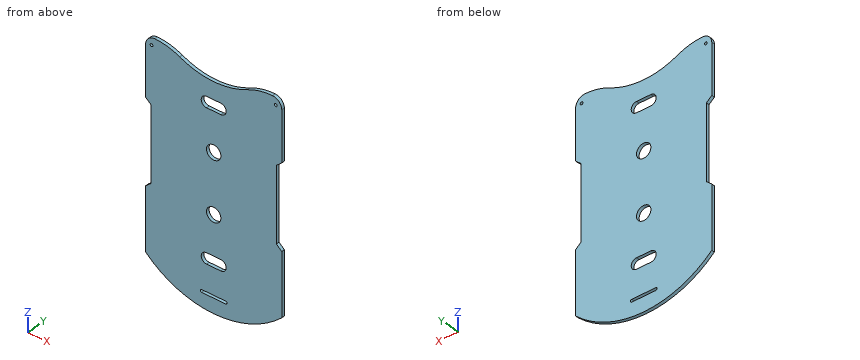
from build123d import *

# Parameters (mm, degrees)
CROQUIS1_R              = 8
CROQUIS1_R_2            = 1.55
SALIENTE_EXTRUIR1_DEPTH = 3.5


with BuildPart() as part:
    # Croquis1 → Saliente-Extruir1 (new body)
    with BuildSketch(Plane(origin=(0, 0, 0), x_dir=(1, 0, 0), z_dir=(0, 1, 0))):
        with BuildLine():
            Line((-75.83, 106.96), (-75.83, 36.96))
            Line((-75.83, 36.96), (-69.88, 31.76))
            Line((-69.88, 31.76), (-69.88, -51.39))
            Line((-69.88, -51.39), (-75.83, -56.59))
            Line((-75.83, -56.59), (-75.83, -112.67))
            ThreePointArc((-75.83, -112.67), (-72.813199846, -119.953199846), (-65.53, -122.97))
            ThreePointArc((-65.53, -122.97), (-51.316231926, -121.339014909), (-37.841336827, -116.530842982))
            ThreePointArc((-37.841336827, -116.530842982), (0, -107.730623626), (37.841336827, -116.530842982))
            ThreePointArc((37.841336827, -116.530842982), (51.316231926, -121.339014909), (65.53, -122.97))
            ThreePointArc((65.53, -122.97), (72.813199846, -119.953199846), (75.83, -112.67))
            Line((75.83, -112.67), (75.83, -56.59))
            Line((75.83, -56.59), (69.88, -51.39))
            Line((69.88, -51.39), (69.88, 31.76))
            Line((69.88, 31.76), (75.83, 36.96))
            Line((75.83, 36.96), (75.83, 106.96))
            ThreePointArc((75.83, 106.96), (0, 137.38), (-75.83, 106.96))
        make_face()
        with Locations(Location((0, 32.92, 0), (0, 0, 270))):
            Circle(CROQUIS1_R, mode=Mode.SUBTRACT)
        with Locations(Location((69.23, -114.59, 0), (0, 0, 270))):
            Circle(CROQUIS1_R_2, mode=Mode.SUBTRACT)
        with Locations(Location((0, -32.92, 0), (0, 0, 90))):
            Circle(CROQUIS1_R, mode=Mode.SUBTRACT)
        with Locations(Location((-69.23, -114.59, 0), (0, 0, 90))):
            Circle(CROQUIS1_R_2, mode=Mode.SUBTRACT)
        with BuildLine():
            Line((-7.895, -88.57), (7.895, -88.57))
            ThreePointArc((7.895, -88.57), (13.91, -82.555), (7.895, -76.54))
            Line((7.895, -76.54), (-7.895, -76.54))
            ThreePointArc((-7.895, -76.54), (-13.91, -82.555), (-7.895, -88.57))
        make_face(mode=Mode.SUBTRACT)
        with BuildLine():
            Line((-7.895, 88.57), (7.895, 88.57))
            ThreePointArc((7.895, 88.57), (13.91, 82.555), (7.895, 76.54))
            Line((7.895, 76.54), (-7.895, 76.54))
            ThreePointArc((-7.895, 76.54), (-13.91, 82.555), (-7.895, 88.57))
        make_face(mode=Mode.SUBTRACT)
        with BuildLine():
            Line((-13.415, 120.93), (13.415, 120.93))
            ThreePointArc((13.415, 120.93), (14.915, 119.43), (13.415, 117.93))
            Line((13.415, 117.93), (-13.415, 117.93))
            ThreePointArc((-13.415, 117.93), (-14.915, 119.43), (-13.415, 120.93))
        make_face(mode=Mode.SUBTRACT)
    extrude(amount=SALIENTE_EXTRUIR1_DEPTH)


solid = part.part
Source: CAD feature listing. Evaluate the final solid. Frame: model axes, mm. Give positions to 0.01 mm unless a question says otherwise; leave off trailing zeros. Write each loop counter-clockwise with the first axis right and the second up, starting at its lowest first coordinate (ties: lowest second). Pieces come first, ordered by that corner, then holes. Notation, with made-up numbers: M 7,21.5 L 25,21.5 A4 cw 25,26.5 Z; hole C 86,85 d6. An arc over 180 degrees is marked long. Answer as a JSON object with one key per item and string values.
Q1. Contact query for flat-ended pins moving along their axis: P1, Ø1.5, axis at x = 17, y = 3, coming from the -Z side; P2, Ø2, axis at x = 6.5, y = 2.5, coming from the +Z side; P3, Ø1.8, axis at y = 1, z = -4.5, coming from the -X side. Output: stop coordinate, or through.
Geometry check:
{"P1": "stops at z = -136.17", "P2": "stops at z = 108.06", "P3": "stops at x = -69.88"}
Q2. Cut plane D-D, the plane x = 47. Return the cut outline in (y, z).
Geometry check:
{"outline": "M 0,-126.8 L 3.5,-126.8 L 3.5,120.17 L 0,120.17 Z"}
Q3. Ray query, line 1 along X through (y, z) = (0.95, 32.92); line 2 along X through (y, z) = (1.9, 114.59); line 3 along Z through (x, y) = (8.5, 1.05). Return the intervals inside material, ascending.
Geometry check:
{"line 1": "x = -69.88 to -8, 8 to 69.88", "line 2": "x = -75.65 to -70.78, -67.68 to -33.61, 33.61 to 67.68, 70.78 to 75.65", "line 3": "z = -137.05 to -120.93, -117.93 to -88.54, -76.57 to 76.57, 88.54 to 108.15"}
Q4. Cut plane C-C, the plane z = 79. Return the cut outline in (x, y).
Geometry check:
{"outline": "M -75.83,0 L -12.75,0 L -12.75,3.5 L -75.83,3.5 Z; M 12.75,0 L 75.83,0 L 75.83,3.5 L 12.75,3.5 Z"}
Q5. Cut plane B-B, the plane y = 1. Count the separate pieces of the cut face and the enclosed holes in it, then the cut area to 3 significant figures.
Geometry check:
{"separate pieces": "1", "enclosed holes": "7", "area": "34,800 mm^2"}
Q6. Cut plane A-A, the plane z = 32.92. Return the cut outline in (x, y), then the cut area to 3 significant figures.
Geometry check:
{"outline": "M -69.88,0 L -8,0 L -8,3.5 L -69.88,3.5 Z; M 8,0 L 69.88,0 L 69.88,3.5 L 8,3.5 Z", "area": "433 mm^2"}
